Can you work these out from the model? Positions are in its coordinate system, mm. Round coordinates to 2 decimals unless told otherwise and drop trailing zeros. Order: outer loops, then holes, each group sorted by start corner. A loop starts at its lowest first (then second) coordinate and runs counter-clockwise, first axis right, second up.
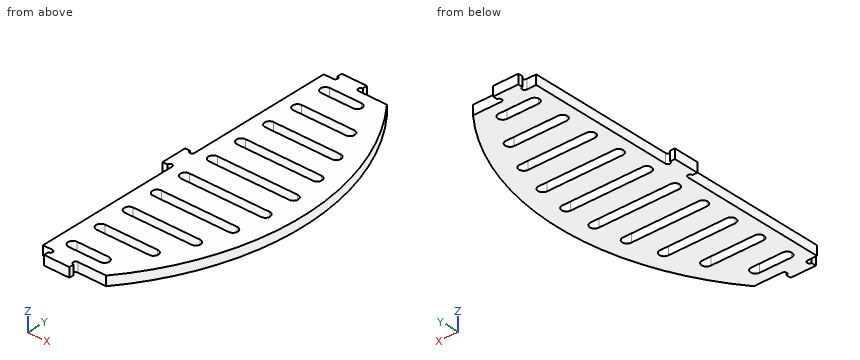
from build123d import *

# Parameters (mm, degrees)
PAD002_DEPTH       = 3
POCKET004_DEPTH    = 3.001
POCKET003006_DEPTH = 3.001


with BuildPart() as part:
    # Sketch006 → Pad002 (new body)
    with BuildSketch(Plane.XY):
        with BuildLine():
            Line((79, -10), (56, -10))
            Line((56, -10), (56, -116))
            Line((56, -116), (79, -116))
            Line((79, -116), (79, -113))
            ThreePointArc((79, -113), (96.55002, -63), (79, -13))
            Line((79, -10), (79, -13))
        make_face()
    extrude(amount=PAD002_DEPTH)

    # Sketch007 → Pocket004 (cut, through all)
    with BuildSketch(Plane.XY.offset(3)):
        with BuildLine():
            Line((79, -10), (70, -10))
            Line((70, -10), (70, -11.498))
            ThreePointArc((70, -11.498), (69.249, -12.249), (70, -13))
            Line((70, -13), (79, -13))
            Line((79, -13), (79, -10))
        make_face()
        with BuildLine():
            Line((62, -13), (59, -13))
            Line((59, -13), (59, -59))
            ThreePointArc((57.498, -59), (58.249, -59.751), (59, -59))
            Line((57.498, -59), (56, -59))
            Line((56, -10), (56, -59))
            Line((62, -10), (56, -10))
            Line((62, -10), (62, -11.498))
            ThreePointArc((62, -13), (62.751, -12.249), (62, -11.498))
        make_face()
        with BuildLine():
            Line((79, -116), (70, -116))
            Line((70, -114.502), (70, -116))
            ThreePointArc((70, -113), (69.249, -113.751), (70, -114.502))
            Line((70, -113), (79, -113))
            Line((79, -113), (79, -116))
        make_face()
        with BuildLine():
            Line((62, -113), (59, -113))
            Line((59, -113), (59, -67))
            ThreePointArc((59, -67), (58.249, -66.249), (57.498, -67))
            Line((56, -67), (57.498, -67))
            Line((56, -67), (56, -116))
            Line((56, -116), (62, -116))
            Line((62, -114.502), (62, -116))
            ThreePointArc((62, -114.502), (62.751, -113.751), (62, -113))
        make_face()
    extrude(amount=-POCKET004_DEPTH, mode=Mode.SUBTRACT)

    # Sketch001006 → Pocket003006 (cut, through all)
    with BuildSketch(Plane.XY.offset(3)):
        with BuildLine():
            Line((64, -109.5), (74.030451, -109.5))
            ThreePointArc((74.030451, -109.5), (75.530451, -108), (74.030451, -106.5))
            Line((64, -106.5), (74.030451, -106.5))
            ThreePointArc((64, -106.5), (62.5, -108), (64, -109.5))
        make_face()
        with BuildLine():
            Line((64, -96.5), (80.61249, -96.5))
            ThreePointArc((80.61249, -99.5), (82.11249, -98), (80.61249, -96.5))
            Line((64, -99.5), (80.61249, -99.5))
            ThreePointArc((64, -96.5), (62.5, -98), (64, -99.5))
        make_face()
        with BuildLine():
            Line((64, -86.5), (85.135733, -86.5))
            ThreePointArc((85.135733, -89.5), (86.635733, -88), (85.135733, -86.5))
            Line((64, -89.5), (85.135733, -89.5))
            ThreePointArc((64, -86.5), (62.5, -88), (64, -89.5))
        make_face()
        with BuildLine():
            Line((64, -76.5), (87.992304, -76.5))
            ThreePointArc((87.992304, -79.5), (89.492304, -78), (87.992304, -76.5))
            Line((64, -79.5), (87.992304, -79.5))
            ThreePointArc((64, -76.5), (62.5, -78), (64, -79.5))
        make_face()
        with BuildLine():
            Line((64, -69.5), (89.378586, -69.5))
            ThreePointArc((89.378586, -69.5), (90.878586, -68), (89.378586, -66.5))
            Line((64, -66.5), (89.378586, -66.5))
            ThreePointArc((64, -66.5), (62.5, -68), (64, -69.5))
        make_face()
        with BuildLine():
            Line((64, -59.5), (89.378586, -59.5))
            ThreePointArc((89.378586, -59.5), (90.878586, -58), (89.378586, -56.5))
            Line((64, -56.5), (89.378586, -56.5))
            ThreePointArc((64, -56.5), (62.5, -58), (64, -59.5))
        make_face()
        with BuildLine():
            Line((64, -49.5), (87.992304, -49.5))
            ThreePointArc((87.992304, -49.5), (89.492304, -48), (87.992304, -46.5))
            Line((64, -46.5), (87.992304, -46.5))
            ThreePointArc((64, -46.5), (62.5, -48), (64, -49.5))
        make_face()
        with BuildLine():
            Line((64, -39.5), (85.135733, -39.5))
            ThreePointArc((85.135733, -39.5), (86.635733, -38), (85.135733, -36.5))
            Line((64, -36.5), (85.135733, -36.5))
            ThreePointArc((64, -36.5), (62.5, -38), (64, -39.5))
        make_face()
        with BuildLine():
            Line((64, -26.5), (80.61249, -26.5))
            ThreePointArc((80.61249, -29.5), (82.11249, -28), (80.61249, -26.5))
            Line((64, -29.5), (80.61249, -29.5))
            ThreePointArc((64, -26.5), (62.5, -28), (64, -29.5))
        make_face()
        with BuildLine():
            Line((64, -16.5), (74.030451, -16.5))
            ThreePointArc((74.030451, -19.5), (75.530451, -18), (74.030451, -16.5))
            Line((64, -19.5), (74.030451, -19.5))
            ThreePointArc((64, -16.5), (62.5, -18), (64, -19.5))
        make_face()
    extrude(amount=-POCKET003006_DEPTH, mode=Mode.SUBTRACT)


solid = part.part
(1) I want a section at B-B, the plane z = 0.6. Give the number of separate pieces and of enclosed holes in the cut face, plus the area to 3 significant figures.
(2) I want a section at A-A, the plane y = -108. List the corners of the cut face in (x, z) for me.
(3) I want a section at D-D, the plane y = -38. List the corners of the cut face in (x, z) for me, plus the area to 3 significant figures.
(4) Please list where these lines run through material, in increasing order: probe 1 along X at (y, z) = (-79, 0.2); probe 2 along X at (y, z) = (-17, 2.35); probe 3 along X at (y, z) = (-62, 2.85).
(5) I'm going to push flat-ended pins straight in: pin 1 Ø1.5 at (x, z) = (79.5, 1.5) entering from -Y; pin 2 Ø1.5 at (x, z) = (60, 1.5) entering from +Y; pin 3 Ø0.7 at (y, z) = (-115, 2) entering from +X. Where does each tip first touch, or does it pass through?
Ans:
1. separate pieces: 1
1. enclosed holes: 10
1. area: 2,610 mm2
2. outline: (59, 0) - (62.5, 0) - (62.5, 3) - (59, 3) - close; (75.53, 0) - (82.69, 0) - (82.69, 3) - (75.53, 3) - close
3. outline: (59, 0) - (62.5, 0) - (62.5, 3) - (59, 3) - close; (86.64, 0) - (92.54, 0) - (92.54, 3) - (86.64, 3) - close
3. area: 28.2 mm2
4. probe 1: x = 59 to 62.88, 89.11 to 94.93
4. probe 2: x = 59 to 62.88, 75.15 to 82
4. probe 3: x = 56 to 96.54
5. pin 1: stops at y = -113
5. pin 2: stops at y = -13
5. pin 3: stops at x = 70
